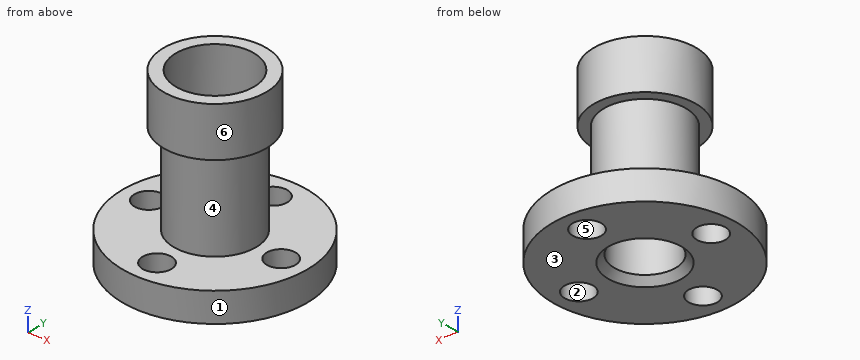
```python
from build123d import *

# Parameters (mm, degrees)
CROQUIS1_R               = 45
SALIENTE_EXTRUIR1_DEPTH  = 14.2
CROQUIS6_R               = 15
SALIENTE_EXTRUIR13_DEPTH = 14
CROQUIS8_R               = 15
CORTAR_EXTRUIR3_DEPTH    = 16
CROQUIS2_R               = 20
SALIENTE_EXTRUIR3_DEPTH  = 58.4
CROQUIS3_R               = 25
CROQUIS3_R_2             = 19
SALIENTE_EXTRUIR4_DEPTH  = 24
CROQUIS5_R               = 15
CORTAR_EXTRUIR4_DEPTH    = 59
CROQUIS7_R               = 7
CORTAR_EXTRUIR18_DEPTH   = 17
CHAFL_N1_SIZE            = 3.5
CHAFL_N1_SIZE2           = 3


with BuildPart() as part:
    # Croquis1 → Saliente-Extruir1 (new body)
    with BuildSketch(Plane.XY):
        Circle(CROQUIS1_R)
    extrude(amount=SALIENTE_EXTRUIR1_DEPTH)

    # Croquis6 → Saliente-Extruir13 (add)
    with BuildSketch(Plane.XY.offset(14.2)):
        Circle(CROQUIS6_R)
    extrude(amount=-SALIENTE_EXTRUIR13_DEPTH)

    # Croquis8 → Cortar-Extruir3 (cut)
    with BuildSketch(Plane.XY.offset(14.2)):
        Circle(CROQUIS8_R)
    extrude(amount=-CORTAR_EXTRUIR3_DEPTH, mode=Mode.SUBTRACT)

    # Croquis2 → Saliente-Extruir3 (add)
    with BuildSketch(Plane.XY):
        Circle(CROQUIS2_R)
    extrude(amount=SALIENTE_EXTRUIR3_DEPTH)

    # Croquis3 → Saliente-Extruir4 (add)
    with BuildSketch(Plane.XY.offset(58.4)):
        Circle(CROQUIS3_R)
        Circle(CROQUIS3_R_2, mode=Mode.SUBTRACT)
    extrude(amount=SALIENTE_EXTRUIR4_DEPTH)

    # Croquis5 → Cortar-Extruir4 (cut)
    with BuildSketch(Plane.XY.offset(58.4)):
        Circle(CROQUIS5_R)
    extrude(amount=-CORTAR_EXTRUIR4_DEPTH, mode=Mode.SUBTRACT)

    # Croquis7 → Cortar-Extruir18 (cut)
    with BuildSketch(Plane(origin=(0, 0, 0), x_dir=(-1, 0, 0), z_dir=(0, 0, -1))):
        with Locations((0, 32.5)):
            Circle(CROQUIS7_R)
        with Locations((32.5, 0)):
            Circle(CROQUIS7_R)
        with Locations((0, -32.5)):
            Circle(CROQUIS7_R)
        with Locations((-32.5, 0)):
            Circle(CROQUIS7_R)
    extrude(amount=-CORTAR_EXTRUIR18_DEPTH, mode=Mode.SUBTRACT)

    # Chaflán1
    chafl_n1_edges = [part.edges().sort_by_distance(p)[0] for p in [
        (-15, 0, 0),
    ]]
    chafl_n1_side = [part.faces().sort_by_distance(p)[0] for p in [
        (-15, 0, 29.2),
    ]]
    chamfer(chafl_n1_edges, length=CHAFL_N1_SIZE, length2=CHAFL_N1_SIZE2, reference=chafl_n1_side[0])


solid = part.part
```
The listing builds one solid part. Answer for the finished solid, in the listing's coordinates (mm). Face numbers are marked on the shaded views. A direction names the side the tool comes from. Coordinates: 2 decimals unless noted, no trailing zeros. Loops run counter-clockwise (first coordinate to the right, second up) from the corner with the lowest first, then second, coordinate; pieces in that order, holes last. Notation, with made-up numbers: (42.25, 59.5) - (99.25, 59.5) arc R14 cw to (99.25, 73.5) - close; hole circle Ø9 at (26.25, -34.75). An arc over 180 degrees is marked (long way). Write item = value, one per line.
1) Section C-C (x = 35.5) is taken. Determine the outline of the cut face in (y, z).
Responses:
outline = (-27.65, 0) - (-6.32, 0) - (-6.32, 14.2) - (-27.65, 14.2) - close; (6.32, 0) - (27.65, 0) - (27.65, 14.2) - (6.32, 14.2) - close
2) Each of these flat-tipped pins is pushed along its axis until it touches: P1, Ø6, axis at y = 6, z = 67.5, coming from the -X side; P2, Ø6, axis at x = 29.5, y = 25, coming from the +Z side; P3, Ø4, axis at y = -28, z = 15, coming from the +X side. Where does it stop, or does it pass through?
Responses:
P1 = -24.82
P2 = 14.2
P3 = 36.61
3) Which of the six approach directions +Z, -Z, +X, -X, +Y, -Y give full straight-line access (tool end or side, diameter ignored) to the marked faces 4, 5 and 6?
Responses:
face_4 = none
face_5 = +Z, -Z
face_6 = +Z
4) Section A-A (y = 0) is taken. Count the separate pieces of the cut face and the enclosed holes in it, plus the area to 3 significant figures.
Responses:
separate_pieces = 4
enclosed_holes = 0
area = 1,170 mm^2
5) Find the intervals of material crossed by line 1 along Y through (x, z) = (0.5, 13.5); line 2 along Y through (x, z) = (0, 73.5); line 3 along Y through (x, z) = (0, 22), in increasing order.
Responses:
line_1 = -45 to -39.48, -25.52 to -14.99, 14.99 to 25.52, 39.48 to 45
line_2 = -25 to -19, 19 to 25
line_3 = -20 to -15, 15 to 20
6) Section B-B (z = 16) is taken. Determine the outline of the cut face in (x, y).
Responses:
outline = circle Ø40 at (0, 0); hole circle Ø30 at (0, 0)
7) Determine the mould class of the marked faces 1, 2 and 3 for opening direction X: pulls with the +X half, pulls with the -X half, needs draft (parallel to the pull), parting line crosses it, or undercut.
Responses:
face_1 = parting line crosses it
face_2 = undercut
face_3 = needs draft
8) Section D-D (y = -36) is taken. Determine the outline of the cut face in (x, z), plus the area to 3 significant figures.
Responses:
outline = (-27, 0) - (-6.06, 0) - (-6.06, 14.2) - (-27, 14.2) - close; (6.06, 0) - (27, 0) - (27, 14.2) - (6.06, 14.2) - close
area = 595 mm^2
